Check sheet for the modelled part. Datum: model origin and axes. Units: mm. A direction names the side the tool comes from. Coordinates: 2 decimals unless noted, no trailing zeros. Loops run counter-clockwise (first coordinate to the right, second up) from the corner with the lowest first, then second, coordinate; pieces in that order, holes last. Notation, with made-up numbers: M 0,45 L 7,45 A12 cw 7,49 Z; hole C 72,25.25 d2. An arc over 180 degrees is marked long. Use CSV: the item, a comma, the result in double quotes. Start each with the question number.
(1) Draft check along Z on faces 1 (the flat face through (0, 0, -24)), 2 (the cylindrical face through (26.274, 5.267, -3.45)), 3 (the cylindrical face through (13.38, 1.48, 25.73)). Enter one of: pulls with the +Z half, pulls with the -Z half, needs draft (parallel to the pull), parting line crosses it, or undercut.
(2) Section check A-A on x = 0. Record the cut outline in (y, z).
(3) Section check D-D on y = 2. Record the cut outline in (x, z).
(4) Section check B-B on z = 7. Record the cut outline in (x, y).
(5) Set-up check for faces 4 (the cylindrical face through (-24.397, 6.451, 12.69)), 5 (the flat face through (14, 10, -23)): record each of +Z, -Z, +X, -X, +Y, -Y from which the full face is reachable in a straight line by a thin tool's end or side.
(6) Section check C-C on y = 5.25. Record the cut outline in (x, z).
(7) Scan lines: line 1 (X direction, y = 0.25, z = 0); line 2 (X direction, y = 8, z = 0); line 3 (Z direction, x = -22, y = 9.25). Record each from-to range of solid material in increasing order.
(8) Go/stop test with flat-tipped pins: pin 1 Ø2 at (y, z) = (3.5, -13.5) entering from -X; pin 2 Ø1.5 at (y, z) = (9, -15.5) entering from -X; pin 3 Ø6 at (y, z) = (3, -8.5) entering from -X. Record where each tip stops, or that it passes through.
from build123d import *

# Parameters (mm, degrees)
SKETCH1_R           = 27.5
BOSS_EXTRUDE1_DEPTH = 10
SKETCH2_R           = 29
SKETCH2_R_2         = 24
EXTRUDE_THIN1_DEPTH = 3
SKETCH3_R           = 26.5
CUT_EXTRUDE1_DEPTH  = 9.6
SKETCH4_R           = 23.5
CUT_EXTRUDE2_DEPTH  = 43.12077872


with BuildPart() as part:
    # Sketch1 → Boss-Extrude1 (new body)
    with BuildSketch(Plane(origin=(0, 0, 0), x_dir=(1, 0, 0), z_dir=(0, 1, 0))):
        with Locations(Location((0, 0, 0), (0, 0, 270))):
            Circle(SKETCH1_R)
    extrude(amount=BOSS_EXTRUDE1_DEPTH)

    # Sketch2 → Extrude-Thin1 (add)
    with BuildSketch(Plane(origin=(0, 0, 0), x_dir=(1, 0, 0), z_dir=(0, 1, 0))):
        Circle(SKETCH2_R)
        Circle(SKETCH2_R_2, mode=Mode.SUBTRACT)
    extrude(amount=EXTRUDE_THIN1_DEPTH)

    # Sketch3 → Cut-Extrude1 (cut)
    with BuildSketch(Plane(origin=(0, 10, 0), x_dir=(1, 0, 0), z_dir=(0, 1, 0))):
        with Locations(Location((0, 0, 0), (0, 0, 270))):
            Circle(SKETCH3_R)
    extrude(amount=-CUT_EXTRUDE1_DEPTH, mode=Mode.SUBTRACT)

    # Sketch4 → Cut-Extrude2 (cut, through all)
    with BuildSketch(Plane(origin=(0, 0.4, 0), x_dir=(1, 0, 0), z_dir=(0, 1, 0))):
        with Locations(Location((0, 0, 0), (0, 0, 270))):
            Circle(SKETCH4_R)
    extrude(amount=-CUT_EXTRUDE2_DEPTH, mode=Mode.SUBTRACT)


solid = part.part
Outcome:
1,face 1,"needs draft"
1,face 2,"undercut"
1,face 3,"parting line crosses it"
2,outline,"M 0,-29 L 3,-29 L 3,-27.5 L 10,-27.5 L 10,-26.5 L 0.4,-26.5 L 0.4,-23.5 L 0,-23.5 Z; M 0,23.5 L 0.4,23.5 L 0.4,26.5 L 10,26.5 L 10,27.5 L 3,27.5 L 3,29 L 0,29 Z"
3,outline,"C 0,0 d58; hole C 0,0 d53"
4,outline,"M -28.14,0 L -22.43,0 L -22.43,0.4 L -25.56,0.4 L -25.56,10 L -26.59,10 L -26.59,3 L -28.14,3 Z; M 22.43,0 L 28.14,0 L 28.14,3 L 26.59,3 L 26.59,10 L 25.56,10 L 25.56,0.4 L 22.43,0.4 Z"
5,face 4,"+Y"
5,face 5,"+Z, -Z, +X, -X, +Y"
6,outline,"C 0,0 d55; hole C 0,0 d53"
7,line 1,"x = -29 to -23.5, 23.5 to 29"
7,line 2,"x = -27.5 to -26.5, 26.5 to 27.5"
7,line 3,"z = -16.5 to -14.77, 14.77 to 16.5"
8,pin 1,"stops at x = -26.1"
8,pin 2,"stops at x = -23.21"
8,pin 3,"stops at x = -28.47"
